```python
from build123d import *

# Parameters (mm, degrees)
BOSS_EXTRUDE1_DEPTH = 101.6
SKETCH2_R           = 2.4638
CUT_EXTRUDE1_DEPTH  = 6.35
SKETCH3_R           = 2.4638
CUT_EXTRUDE2_DEPTH  = 6.35


with BuildPart() as part:
    # Sketch1 → Boss-Extrude1 (new body)
    with BuildSketch(Plane.XY):
        Polygon((0, 0), (0, 47.625), (-3.175, 47.625), (-3.175, -3.175), (47.625, -3.175), (47.625, 0), align=None)
    extrude(amount=BOSS_EXTRUDE1_DEPTH)

    # Sketch2 → Cut-Extrude1 (cut)
    with BuildSketch(Plane(origin=(0, 0, 0), x_dir=(1, 0, 0), z_dir=(0, 1, 0))):
        with Locations((25.4, -76.2)):
            Circle(SKETCH2_R)
        with Locations((25.4, -25.4)):
            Circle(SKETCH2_R)
    extrude(amount=-CUT_EXTRUDE1_DEPTH, mode=Mode.SUBTRACT)

    # Sketch3 → Cut-Extrude2 (cut)
    with BuildSketch(Plane(origin=(0, 0, 0), x_dir=(0, 0, -1), z_dir=(1, 0, 0))):
        with Locations((-25.4, 22.225)):
            Circle(SKETCH3_R)
        with Locations((-76.2, 22.225)):
            Circle(SKETCH3_R)
    extrude(amount=-CUT_EXTRUDE2_DEPTH, mode=Mode.SUBTRACT)


solid = part.part
```
Geometry check sheet. Reference: the model listing, model coordinates, mm. A direction names the side the tool comes from. Round coordinates to 2 decimals unless told otherwise and drop trailing zeros. Order: outer loops, then holes, each group sorted by start corner. A loop starts at its lowest first (then second) coordinate and runs counter-clockwise, first axis right, second up. Notation, with made-up numbers: (48.25, 17) -> (101.25, 17) arc R16 cw to (101.25, 27) -> close; hole circle Ø8 at (46, -32). An arc over 180 degrees is marked (long way). Return JSON: item names as keys, results as strings. Group by question number.
Q1. Tool access check on faces 1 (the flat face through (24, 0, 50)), 2 (the cylindrical face through (-1.565, 23.89, 27.216)). Record the directions out of +Z, -Z, +X, -X, +Y, -Y that give a thin tool (end or side, any length) a straight path to the whole face; none if there is none.
Q2. Gauge pin test, flat ends, axial feed: pin 1 (6 mm diameter, centred on y = 30, z = 41, fed in from +X); pin 2 (10 mm diameter, centred on x = 15, z = 50.5, fed in from +Y). Record the tip position at first contact, or that the pin passes through.
Q3. Section check A-A, the plane x = 25.4. Record the boundary of the cut face in (y, z) (3 decimals), plus the area to 3 significant figures.
Q4. Material ranges on probe 1 along Y at (x, z) = (-0.95, 76.2) (3 decimals); probe 2 along Y at (x, z) = (15, 51.5) (3 decimals); probe 3 along Z at (x, y) = (25, -1), recorded low to high. Write a range as from..to.
Q5. Section check D-D, the plane y = 11.5. Record the boundary of the cut face in (x, z) (3 decimals).
Q6. Section check B-B, the plane z = 76.2. Record the boundary of the cut face in (x, y) (3 decimals), plus the area to 3 significant figures.
Q7. Section check C-C, the plane z = 17.5. Record the boundary of the cut face in (x, y) (3 decimals).
Q8. Release check for a two-part mould opening along Z. For faces 3 (the flat face through (22, -3.175, 50)), 4 (the cylindrical face through (26.72, -1.57, 23.32)), 5 (the flat face through (-0.5, 11.1, 0)) record: released by +Z, released by -Z, zero draft, split by the parting line, or undercut.
Numbers:
{
 "1": {"face 1": "+Z, -Z, +X, +Y", "face 2": "+X, -X"},
 "2": {"pin 1": "x = 0", "pin 2": "y = 0"},
 "3": {"outline": "(-3.175, 0) -> (0, 0) -> (0, 22.936) -> (-3.175, 22.936) -> close; (-3.175, 27.864) -> (0, 27.864) -> (0, 73.736) -> (-3.175, 73.736) -> close; (-3.175, 78.664) -> (0, 78.664) -> (0, 101.6) -> (-3.175, 101.6) -> close", "area": "291 mm^2"},
 "4": {"probe 1": "-3.175..19.761, 24.689..47.625", "probe 2": "-3.175..0", "probe 3": "0..22.97, 27.83..73.77, 78.63..101.6"},
 "5": {"outline": "(-3.175, 0) -> (0, 0) -> (0, 101.6) -> (-3.175, 101.6) -> close"},
 "6": {"outline": "(-3.175, -3.175) -> (22.936, -3.175) -> (22.936, 0) -> (0, 0) -> (0, 19.761) -> (-3.175, 19.761) -> close; (-3.175, 24.689) -> (0, 24.689) -> (0, 47.625) -> (-3.175, 47.625) -> close; (27.864, -3.175) -> (47.625, -3.175) -> (47.625, 0) -> (27.864, 0) -> close", "area": "281 mm^2"},
 "7": {"outline": "(-3.175, -3.175) -> (47.625, -3.175) -> (47.625, 0) -> (0, 0) -> (0, 47.625) -> (-3.175, 47.625) -> close"},
 "8": {"face 3": "zero draft", "face 4": "undercut", "face 5": "released by -Z"}
}
